Here's how the part is built. I have some questions about the finished solid (model axes, mm). A direction names the side the tool comes from. Round coordinates to 2 decimals unless told otherwise and drop trailing zeros. Loops run counter-clockwise (first coordinate to the right, second up) from the corner with the lowest first, then second, coordinate; pieces in that order, holes last. Notation, with made-up numbers: M 43.25,78.25 L 101.25,78.25 A27 cw 101.25,98.25 Z; hole C -24,33 d5. An arc over 180 degrees is marked long. Answer as a JSON object with one key per item and string values.
from build123d import *

# Parameters (mm, degrees)
BOSS_EXTRUDE1_DEPTH      = 8
SKETCH2_W                = 3
SKETCH2_H                = 6
CUT_EXTRUDE1_DEPTH       = 16
CUT_EXTRUDE2_START       = -7
CUT_EXTRUDE2_OUTLINE_R   = 1
CUT_EXTRUDE2_OUTLINE_R_2 = 1.25
CUT_EXTRUDE2_DEPTH       = 7
SKETCH4_R                = 11.300905521
SKETCH4_R_2              = 4
CUT_EXTRUDE3_DEPTH       = 3
SKETCH5_W                = 0.851480407
SKETCH5_H                = 4
CUT_EXTRUDE4_DEPTH       = 8
CUT_EXTRUDE5_DEPTH       = 1
CUT_EXTRUDE5_DEPTH_BACK  = 2
SKETCH6_R                = 2.5


# Read off the part's stored shape, not the designer's step: Cut-Extrude2
with BuildPart() as part:
    # Sketch1 → Boss-Extrude1 (new, symmetric)
    with BuildSketch(Plane(origin=(0, 0, 0), x_dir=(0, 0, -1), z_dir=(1, 0, 0))):
        Polygon((0, -5), (0, 5), (-4, 5), (-4, 4), (-7, 4), (-7, -4), (-4, -4), (-4, -5), align=None)
    extrude(amount=BOSS_EXTRUDE1_DEPTH, both=True)

    # Sketch2 → Cut-Extrude1 (cut)
    with BuildSketch(Plane.ZY.offset(8)):
        with Locations((3.5, 0)):
            Rectangle(SKETCH2_W, SKETCH2_H)
    extrude(amount=-CUT_EXTRUDE1_DEPTH, mode=Mode.SUBTRACT)

    # Cut-Extrude2 outline → Cut-Extrude2 (cut)
    with BuildSketch(Plane.XY.offset(7).offset(CUT_EXTRUDE2_START)):
        with BuildLine():
            ThreePointArc((-8.000004764, 0), (-7.481459456, 2.692583288), (-6, 5))
            Line((-6, 5), (-8, 5))
            Line((-8, 5), (-8.000004764, 0))
        make_face()
        with BuildLine():
            ThreePointArc((-6, -5), (-7.481459456, -2.692583288), (-8.000004764, 0))
            Line((-8.000004764, 0), (-8, -5))
            Line((-8, -5), (-6, -5))
        make_face()
        with BuildLine():
            Line((8, 5), (6, 5))
            ThreePointArc((6, 5), (7.481456009, 2.692582404), (8, 0))
            Line((8, 0), (8, 5))
        make_face()
        with BuildLine():
            Line((8, -5), (8, 0))
            ThreePointArc((8, 0), (7.481456009, -2.692582404), (6, -5))
            Line((6, -5), (8, -5))
        make_face()
        with Locations((-6, 0)):
            Circle(CUT_EXTRUDE2_OUTLINE_R)
        Circle(CUT_EXTRUDE2_OUTLINE_R_2)
        with Locations((6, 0)):
            Circle(CUT_EXTRUDE2_OUTLINE_R)
    extrude(amount=CUT_EXTRUDE2_DEPTH, mode=Mode.SUBTRACT)

    # Sketch4 → Cut-Extrude3 (cut)
    with BuildSketch(Plane.XY.offset(7)):
        Circle(SKETCH4_R)
        Circle(SKETCH4_R_2, mode=Mode.SUBTRACT)
    extrude(amount=-CUT_EXTRUDE3_DEPTH, mode=Mode.SUBTRACT)

    # Sketch5 → Cut-Extrude4 (cut, symmetric)
    with BuildSketch(Plane(origin=(0, 0, 0), x_dir=(0, 0, -1), z_dir=(1, 0, 0))):
        with Locations((-6.574259796, 0)):
            Rectangle(SKETCH5_W, SKETCH5_H)
    extrude(amount=CUT_EXTRUDE4_DEPTH, both=True, mode=Mode.SUBTRACT)

    # Sketch6 → Cut-Extrude5 (cut, two sides: drawn at the far end of the back side and taken through both)
    with BuildSketch(Plane.XY.offset(6.148519593).offset(-CUT_EXTRUDE5_DEPTH_BACK)):
        with Locations(Location((0, 0, 0), (0, 0, 233.130102354))):
            Circle(SKETCH6_R)
    extrude(amount=CUT_EXTRUDE5_DEPTH + CUT_EXTRUDE5_DEPTH_BACK, mode=Mode.SUBTRACT)


solid = part.part
Item 1: I want a section at D-D on y = 1.5. List the corners of the cut face in (x, z) for me, plus the area to 3 significant figures.
Solution:
{"outline": "M -7.84,0 L 7.84,0 L 7.84,2 L -7.84,2 Z; M -3.71,5 L -2,5 L -2,6.15 L -3.71,6.15 Z; M 2,5 L 3.71,5 L 3.71,6.15 L 2,6.15 Z", "area": "35.3 mm2"}
Item 2: We'd pull the mould along Y, two halves only. Please class faces 4 (the face through (0, -3, 3)), 5 (the face through (0, 5, 2)), 6 (the face through (2.5, -2, 6.6)), 7 (the face through (0.1, 4.2, 4)): +Y half, -Y half, draft (parallel to the pull), parting line (faces both ways), or undercut.
Solution:
{"face 4": "undercut", "face 5": "+Y half", "face 6": "undercut", "face 7": "draft"}
Item 3: For faces 1 (the face through (2.5, 2, 6.6)), 2 (the face through (-3, 0, 5)), 3 (the face through (-0.1, -4.2, 4)), which set-ups out of +Z, -Z, +X, -X, +Y, -Y let a thin tool reach every point of the face, with its end or its side?
Solution:
{"face 1": "+Z, +X, -X", "face 2": "+X, -X", "face 3": "+Z, -Y"}
Item 4: I want a section at B-B on x = -6.75. List the corners of the cut face in (y, z) for me, plus the area to 3 significant figures.
Solution:
{"outline": "M -4.07,0 L -0.66,0 L -0.66,2 L -3,2 L -3,4 L -4.07,4 Z; M 0.66,0 L 4.07,0 L 4.07,4 L 3,4 L 3,2 L 0.66,2 Z", "area": "17.9 mm2"}
Item 5: I want a section at A-A on z = 3.5. List the corners of the cut face in (x, y) for me.
Solution:
{"outline": "M -7.35,-3 A7.25 ccw -6,-5 L 6,-5 A7.25 ccw 7.35,-3 Z; M -7.35,3 L 7.35,3 A7.25 ccw 6,5 L -6,5 A7.25 ccw Z"}
Item 6: For P1, Ø4, axis at x = 0, y = 0, coming from the +Z side; P2, Ø1, axis at x = 3.5, y = 4.5, coming from the +Z side; P3, Ø0.9, axis at x = 3, z = 6.5, coming from the -Y side, each with a flat end and sliding along its axis, tell me the tip position at first contact or that it passes through.
Solution:
{"P1": "stops at z = 2", "P2": "stops at z = 4", "P3": "stops at y = -3.08"}
Item 7: I want a section at C-C on z = 1.5. Count the separate pieces of the cut face and the enclosed holes in it, plus the area to 3 significant figures.
Solution:
{"separate pieces": "1", "enclosed holes": "3", "area": "136 mm2"}
Item 8: If I drill on L1, parallel to X at y = 0, z = 6.1; L2, parallel to Y at x = 0, z = 0.65, over which ranges is the centre line in solid material (lowest first)? Write a range as from..to.
Solution:
{"L1": "x = -4..-2.5, 2.5..4", "L2": "y = -5..-1.25, 1.25..5"}
